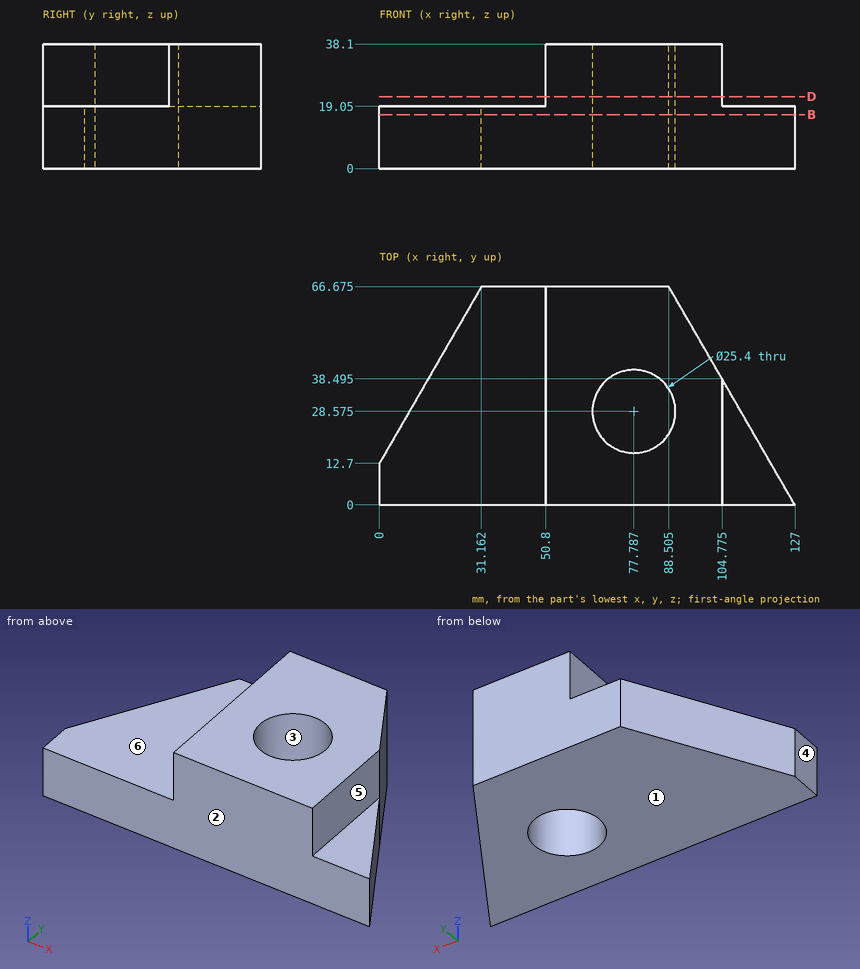
Can you work these out from the drawing? Everything is in mm from the part's minimum corner. A direction names the side the tool comes from. Coordinates: 2 decimals unless noted, no trailing zeros. Loops run counter-clockwise (first coordinate to the right, second up) from the corner with the lowest first, then second, coordinate; pieces in that order, holes last. Notation, with made-up numbers: (24.5, -8.75) - (51.5, -8.75) arc R13 ccw to (51.5, 8.25) - close; hole circle Ø4 at (47, -17). An arc over 180 degrees is marked (long way). Put each result on its own line as item: value. Start each with the question number.
Item 1: Suppose I cut it at D-D (z = 22). Please give me the cut outline in (x, y) (1 decimal).
Item 2: If we mould it in two halves opening along Y, with no side actions, what happens to the marked faces 1, 2 and 3? For each: +Y half, -Y half, draft (parallel to the pull), parting line (faces both ways), or undercut.
Item 3: If I drill on line 1 along X through (y, z) = (29, 28) (1 decimal); line 2 along X through (y, z) = (15.5, 29) (1 decimal); line 3 along Z through (x, y) = (18, 36), over which ranges is the centre line in solid material (lowest first)?
Item 4: Suppose I cut it at B-B (z = 16.5). Please give me the cut outline in (x, y) (1 decimal).
Item 5: Which directions (+Z, -Z, +X, -X, +Y, -Y) give clear straight access to the entire face, cutting with the end or side of a thin tool? Please do the marked faces 4, 5 and 6.
Item 6: For pin 1 (4 mm diameter, centred on x = 18.5, z = 20, fed in from +Y); pin 2 (1.5 mm diameter, centred on y = 52.5, z = 33.5, fed in from +X); pin 3 (5 mm diameter, centred on y = 38, z = 17, fed in from +X) (1 decimal), each with a flat end and sliding along its axis, tell me the tip position at first contact or that it passes through.
Here are the results:
1. outline: (50.8, 0) - (104.8, 0) - (104.8, 38.5) - (88.5, 66.7) - (50.8, 66.7) - close; hole circle Ø25.4 at (77.8, 28.6)
2. face 1: draft
2. face 2: -Y half
2. face 3: undercut
3. line 1: 50.8 to 65.1, 90.5 to 104.8
3. line 2: 50.8 to 104.8
3. line 3: 0 to 19.05
4. outline: (0, 0) - (127, 0) - (88.5, 66.7) - (31.2, 66.7) - (0, 12.7) - close; hole circle Ø25.4 at (77.8, 28.6)
5. face 4: +Z, -Z, -X, +Y, -Y
5. face 5: +Z, +X, +Y, -Y
5. face 6: +Z, -X, +Y, -Y
6. pin 1: y = 47.79
6. pin 2: x = 97.12
6. pin 3: x = 106.5
